```python
from build123d import *

# Parameters (mm, degrees)
SKETCH2_W                = 200
SKETCH2_H                = 150
BOSS_EXTRUDE1_DEPTH      = 80
FILLET1_R                = 10
SHELL1_T                 = -2
SHELL1_THICKNESS_2_DEPTH = 13
SKETCH5_W                = 2
SKETCH5_H                = 4
CUT_EXTRUDE1_DEPTH       = 2
BOSS_EXTRUDE2_DEPTH      = 16
SKETCH7_W                = 36.5
SKETCH7_H                = 27.5
CUT_EXTRUDE2_DEPTH       = 2
BOSS_EXTRUDE3_DEPTH      = 16
SKETCH10_W               = 36.5
SKETCH10_H               = 27.5
CUT_EXTRUDE4_DEPTH       = 2
BOSS_EXTRUDE4_DEPTH      = 16
SKETCH13_W               = 38
SKETCH13_H               = 19.1
CUT_EXTRUDE5_DEPTH       = 2
BOSS_EXTRUDE5_DEPTH      = 13.5
SKETCH15_W               = 10.5
SKETCH15_H               = 9.367949192
CUT_EXTRUDE6_DEPTH       = 3
CUT_EXTRUDE8_REACH       = 150.408
SKETCH20_R               = 8
SPLIT1_SURFACE_1_BACK    = 263.488
SPLIT1_SURFACE_1_DEPTH   = 526.976
SPLIT1_SURFACE_2_BACK    = 263.488
SPLIT1_SURFACE_2_DEPTH   = 526.976
SPLIT2_SURFACE_3_BACK    = 263.488
SPLIT2_SURFACE_3_DEPTH   = 526.976
SPLIT2_SURFACE_4_BACK    = 263.488
SPLIT2_SURFACE_4_DEPTH   = 526.976


with BuildPart() as part:
    # Sketch2 → Boss-Extrude1 (new body)
    with BuildSketch(Plane(origin=(0, 0, 0), x_dir=(1, 0, 0), z_dir=(0, 1, 0))):
        Rectangle(SKETCH2_W, SKETCH2_H)
    extrude(amount=BOSS_EXTRUDE1_DEPTH)

    # Fillet1
    fillet1_edges = [part.edges().sort_by_distance(p)[0] for p in [
        (100, 40, 75),
        (-100, 40, 75),
        (-100, 40, -75),
        (100, 40, -75),
    ]]
    fillet(fillet1_edges, radius=FILLET1_R)

    # Shell1
    shell1_openings = [part.faces().sort_by_distance(p)[0] for p in [
        (0, 80, 0),
    ]]
    offset(amount=SHELL1_T, openings=shell1_openings, kind=Kind.INTERSECTION)

    # Shell1 thickness 2 face (on inner face of the shell) → Shell1 thickness 2 (add)
    with BuildSketch(Plane(origin=(0, 2, 0), x_dir=(0, 0, -1), z_dir=(0, -1, 0))):
        with BuildLine():
            ThreePointArc((73, -90), (70.656854249, -95.656854249), (65, -98))
            Line((65, -98), (-65, -98))
            ThreePointArc((-65, -98), (-70.656854249, -95.656854249), (-73, -90))
            Line((-73, -90), (-73, 90))
            ThreePointArc((-73, 90), (-70.656854249, 95.656854249), (-65, 98))
            Line((-65, 98), (65, 98))
            ThreePointArc((65, 98), (70.656854249, 95.656854249), (73, 90))
            Line((73, 90), (73, -90))
        make_face()
    extrude(amount=-SHELL1_THICKNESS_2_DEPTH)

    # Sketch5 → Cut-Extrude1 (cut)
    with BuildSketch(Plane.XY.offset(75)):
        Polygon((18.25, 44.5), (-18.25, 44.5), (-18.25, 40.5), (-18.25, 21), (-18.25, 17), (18.25, 17), (18.25, 21), (18.25, 40.5), align=None)
        with Locations((-19.25, 42.5)):
            Rectangle(SKETCH5_W, SKETCH5_H)
        with Locations((19.25, 42.5)):
            Rectangle(SKETCH5_W, SKETCH5_H)
        with Locations((-19.25, 19)):
            Rectangle(SKETCH5_W, SKETCH5_H)
        with Locations((19.25, 19)):
            Rectangle(SKETCH5_W, SKETCH5_H)
    extrude(amount=-CUT_EXTRUDE1_DEPTH, mode=Mode.SUBTRACT)

    # Sketch6 → Boss-Extrude2 (add)
    with BuildSketch(Plane(origin=(0, 0, 73), x_dir=(-1, 0, 0), z_dir=(0, 0, -1))):
        Polygon((18.25, 15), (22.25, 15), (22.25, 47.5), (18.25, 47.5), (18.25, 44.5), (20.25, 44.5), (20.25, 40.5), (18.25, 40.5), (18.25, 21), (20.25, 21), (20.25, 17), (18.25, 17), align=None)
        Polygon((-22.25, 47.5), (-22.25, 15), (-18.25, 15), (-18.25, 17), (-20.25, 17), (-20.25, 21), (-18.25, 21), (-18.25, 40.5), (-20.25, 40.5), (-20.25, 44.5), (-18.25, 44.5), (-18.25, 47.5), align=None)
    extrude(amount=BOSS_EXTRUDE2_DEPTH)

    # Sketch7 → Cut-Extrude2 (cut)
    with BuildSketch(Plane(origin=(100, 0, 0), x_dir=(0, 0, -1), z_dir=(1, 0, 0))):
        with Locations((0, 30.75)):
            Rectangle(SKETCH7_W, SKETCH7_H)
        Polygon((-18.25, 43.5), (-19.75, 44.366025404), (-19.75, 41.633974596), (-18.25, 42.5), align=None)
        Polygon((-19.75, 19.866025404), (-18.25, 19), (-18.25, 18), (-19.75, 17.133974596), align=None)
        Polygon((19.75, 17.133974596), (19.75, 19.866025404), (18.25, 19), (18.25, 18), align=None)
        Polygon((19.75, 41.633974596), (18.25, 42.5), (18.25, 43.5), (19.75, 44.366025404), align=None)
    extrude(amount=-CUT_EXTRUDE2_DEPTH, mode=Mode.SUBTRACT)

    # Sketch8 → Boss-Extrude3 (add)
    with BuildSketch(Plane.ZY.offset(-98)):
        Polygon((-21.25, 47.5), (-18.25, 47.5), (-18.25, 43.5), (-19.75, 44.366025404), (-19.75, 41.633974596), (-18.25, 42.5), (-18.25, 19), (-19.75, 19.866025404), (-19.75, 17.133974596), (-18.25, 18), (-18.25, 15), (-21.25, 15), align=None)
        Polygon((19.75, 44.366025404), (18.25, 43.5), (18.25, 47.5), (21.25, 47.5), (21.25, 15), (18.25, 15), (18.25, 18), (19.75, 17.133974596), (19.75, 19.866025404), (18.25, 19), (18.25, 42.5), (19.75, 41.633974596), align=None)
    extrude(amount=BOSS_EXTRUDE3_DEPTH)

    # Sketch10 → Cut-Extrude4 (cut)
    with BuildSketch(Plane.ZY.offset(100)):
        with Locations((0, 30.75)):
            Rectangle(SKETCH10_W, SKETCH10_H)
        Polygon((-18.25, 43.5), (-19.75, 44.366025404), (-19.75, 41.633974596), (-18.25, 42.5), align=None)
        Polygon((-19.75, 19.866025404), (-18.25, 19), (-18.25, 18), (-19.75, 17.133974596), align=None)
        Polygon((19.75, 17.133974596), (19.75, 19.866025404), (18.25, 19), (18.25, 18), align=None)
        Polygon((19.75, 41.633974596), (18.25, 42.5), (18.25, 43.5), (19.75, 44.366025404), align=None)
    extrude(amount=-CUT_EXTRUDE4_DEPTH, mode=Mode.SUBTRACT)

    # Sketch11 → Boss-Extrude4 (add)
    with BuildSketch(Plane(origin=(-98, 0, 0), x_dir=(0, 0, -1), z_dir=(1, 0, 0))):
        Polygon((-18.25, 47.5), (-21.25, 47.5), (-21.25, 15), (-18.25, 15), (-18.25, 18), (-19.75, 17.133974596), (-19.75, 19.866025404), (-18.25, 19), (-18.25, 42.5), (-19.75, 41.633974596), (-19.75, 44.366025404), (-18.25, 43.5), align=None)
        Polygon((19.75, 44.366025404), (18.25, 43.5), (18.25, 47.5), (21.25, 47.5), (21.25, 15), (18.25, 15), (18.25, 18), (19.75, 17.133974596), (19.75, 19.866025404), (18.25, 19), (18.25, 42.5), (19.75, 41.633974596), align=None)
    extrude(amount=BOSS_EXTRUDE4_DEPTH)

    # Sketch13 → Cut-Extrude5 (cut)
    with BuildSketch(Plane.XY.offset(75)):
        Polygon((41, 39.3), (39.5, 40.166025404), (39.5, 37.433974596), (41, 38.3), align=None)
        with Locations((60, 30.75)):
            Rectangle(SKETCH13_W, SKETCH13_H)
        Polygon((41, 22.2), (39.5, 21.333974596), (39.5, 24.066025404), (41, 23.2), align=None)
        Polygon((79, 22.2), (79, 23.2), (80.5, 24.066025404), (80.5, 21.333974596), align=None)
        Polygon((79, 39.3), (80.5, 40.166025404), (80.5, 37.433974596), (79, 38.3), align=None)
    extrude(amount=-CUT_EXTRUDE5_DEPTH, mode=Mode.SUBTRACT)

    # Sketch14 → Boss-Extrude5 (add)
    with BuildSketch(Plane(origin=(0, 0, 73), x_dir=(-1, 0, 0), z_dir=(0, 0, -1))):
        Polygon((-79, 43.3), (-82, 43.3), (-82, 15), (-79, 15), (-79, 22.2), (-80.5, 21.333974596), (-80.5, 24.066025404), (-79, 23.2), (-79, 38.3), (-80.5, 37.433974596), (-80.5, 40.166025404), (-79, 39.3), align=None)
        Polygon((-39.5, 40.166025404), (-41, 39.3), (-41, 43.3), (-38, 43.3), (-38, 15), (-41, 15), (-41, 22.2), (-39.5, 21.333974596), (-39.5, 24.066025404), (-41, 23.2), (-41, 38.3), (-39.5, 37.433974596), align=None)
    extrude(amount=BOSS_EXTRUDE5_DEPTH)

    # Sketch15 → Cut-Extrude6 (cut)
    with BuildSketch(Plane.ZY.offset(-38)):
        with Locations((66.75, 30.75)):
            Rectangle(SKETCH15_W, SKETCH15_H)
    extrude(amount=-CUT_EXTRUDE6_DEPTH, mode=Mode.SUBTRACT)

    # Sketch18 → Cut-Revolve1 (revolve, cut)
    with BuildSketch(Plane(origin=(0, 0, 0), x_dir=(0, 0, -1), z_dir=(1, 0, 0)), mode=Mode.PRIVATE) as cut_revolve1_sk:
        Polygon((-42.5, 0), (-70, 0), (-47.5, 10), (-42.5, 10), align=None)
    revolve(cut_revolve1_sk.sketch.rotate(Axis((0, 0, 0), (0, 1, 0)), 180), axis=Axis((0, 0, 0), (0, 1, 0)), mode=Mode.SUBTRACT)

    # Cut-Extrude8: up to this face of the body (flat: up to its plane)
    cut_extrude8_end = Plane(part.part.faces().sort_by_distance((-0.172584848, 15, -0.486016332))[0])
    # Sketch20 → Cut-Extrude8 (cut, up to the picked face)
    with BuildSketch(Plane.XZ, mode=Mode.PRIVATE) as cut_extrude8_sk1:
        with Locations(Location((0, -42.5, 0), (0, 0, 270))):
            Circle(SKETCH20_R)
    cut_extrude8_tool1 = split(extrude(cut_extrude8_sk1.sketch, amount=-CUT_EXTRUDE8_REACH, mode=Mode.PRIVATE), bisect_by=cut_extrude8_end, keep=Keep.BOTH, mode=Mode.PRIVATE)
    add(cut_extrude8_tool1.solids().sort_by(Axis((0, 0, -42.5), (0, 1, 0)))[0], mode=Mode.SUBTRACT)


with BuildPart() as body_2:
    # Split1: the piece behind the surface
    add(part.part)
    # Split1 surface: a surface, the sketch's curves swept straight by 526.976 mm
    with BuildLine(Plane.XY.offset(75).offset(-SPLIT1_SURFACE_1_BACK), mode=Mode.PRIVATE) as split1_surface_1_path:
        Line((-23.25, 49.5), (23.25, 49.5))
        Line((23.25, 49.5), (23.25, 12))
        Line((23.25, 12), (-23.25, 12))
        Line((-23.25, 12), (-23.25, 49.5))
    split1_surface_1 = Shell.extrude(split1_surface_1_path.wire(), (0 * SPLIT1_SURFACE_1_DEPTH, 0 * SPLIT1_SURFACE_1_DEPTH, 1 * SPLIT1_SURFACE_1_DEPTH))
    split(bisect_by=split1_surface_1, keep=Keep.BOTTOM)


with BuildPart() as part_1:
    add(part.part)

    # Split1: split by a surface, the side it looks to stays
    # Split1 surface: a surface, the sketch's curves swept straight by 526.976 mm
    with BuildLine(Plane.XY.offset(75).offset(-SPLIT1_SURFACE_2_BACK), mode=Mode.PRIVATE) as split1_surface_2_path:
        Line((-23.25, 49.5), (23.25, 49.5))
        Line((23.25, 49.5), (23.25, 12))
        Line((23.25, 12), (-23.25, 12))
        Line((-23.25, 12), (-23.25, 49.5))
    split1_surface_2 = Shell.extrude(split1_surface_2_path.wire(), (0 * SPLIT1_SURFACE_2_DEPTH, 0 * SPLIT1_SURFACE_2_DEPTH, 1 * SPLIT1_SURFACE_2_DEPTH))
    split(bisect_by=split1_surface_2, keep=Keep.TOP)


with BuildPart() as body_3:
    # Split2: the piece behind the surface
    add(body_2.part)
    # Split2 surface: a surface, the sketch's curves swept straight by 526.976 mm
    with BuildLine(Plane(origin=(0, 15, 0), x_dir=(1, 0, 0), z_dir=(0, 1, 0)).offset(-SPLIT2_SURFACE_3_BACK), mode=Mode.PRIVATE) as split2_surface_3_path:
        Line((-23.25, -75), (23.25, -75))
        Line((23.25, -75), (23.25, -50))
        Line((23.25, -50), (-23.25, -50))
        Line((-23.25, -50), (-23.25, -75))
    split2_surface_3 = Shell.extrude(split2_surface_3_path.wire(), (0 * SPLIT2_SURFACE_3_DEPTH, 1 * SPLIT2_SURFACE_3_DEPTH, 0 * SPLIT2_SURFACE_3_DEPTH))
    split(bisect_by=split2_surface_3, keep=Keep.BOTTOM)


with BuildPart() as body_2_1:
    add(body_2.part)

    # Split2: split by a surface, the side it looks to stays
    # Split2 surface: a surface, the sketch's curves swept straight by 526.976 mm
    with BuildLine(Plane(origin=(0, 15, 0), x_dir=(1, 0, 0), z_dir=(0, 1, 0)).offset(-SPLIT2_SURFACE_4_BACK), mode=Mode.PRIVATE) as split2_surface_4_path:
        Line((-23.25, -75), (23.25, -75))
        Line((23.25, -75), (23.25, -50))
        Line((23.25, -50), (-23.25, -50))
        Line((-23.25, -50), (-23.25, -75))
    split2_surface_4 = Shell.extrude(split2_surface_4_path.wire(), (0 * SPLIT2_SURFACE_4_DEPTH, 1 * SPLIT2_SURFACE_4_DEPTH, 0 * SPLIT2_SURFACE_4_DEPTH))
    split(bisect_by=split2_surface_4, keep=Keep.TOP)


solid = body_2_1.part
```
Design review of the part built by this model. Coordinates are the model's own, in mm. A direction names the side the tool comes from. Give positions to 0.01 mm unless a question says otherwise; leave off trailing zeros. Write each loop counter-clockwise with the first axis right and the second up, starting at its lowest first coordinate (ties: lowest second). Pieces come first, ordered by that corner, then holes.
(1) Add section D-D (z = 54.25). Give the boundary of the cut face in (x, y).
Checked values:
outline: (-23.25, 12) - (23.25, 12) - (23.25, 15) - (-23.25, 15) - close
(2) Wall thickness on line 1 along Y through (x, z) = (-19.5, 68); line 2 along X through (y, z) = (40, 72); line 3 along X through (y, z) = (42, 70.75): over which ranges is each line inside the solid? List them lowest first.
Checked values:
line 1: y = 12 to 17, 21 to 40.5, 44.5 to 47.5
line 2: x = -22.25 to -18.25, 18.25 to 22.25
line 3: x = -22.25 to -20.25, 20.25 to 22.25
(3) Add section A-A (y = 29). Give the boundary of the cut face in (x, z).
Checked values:
outline: (-23.25, 73) - (-22.25, 73) - (-22.25, 57) - (-18.25, 57) - (-18.25, 75) - (-23.25, 75) - close; (18.25, 57) - (22.25, 57) - (22.25, 73) - (23.25, 73) - (23.25, 75) - (18.25, 75) - close
(4) Add section B-B (x = -3). Give the boundary of the cut face in (y, z), and give its area (3 significant figures).
Checked values:
outline: (12, 50) - (15, 50) - (15, 73) - (17, 73) - (17, 75) - (12, 75) - close; (44.5, 73) - (49.5, 73) - (49.5, 75) - (44.5, 75) - close
area: 89.0 mm2
(5) Tool access review of faces 1 (the face through (20.25, 42, 66)), 2 (the face through (-18.25, 16, 65)), 3 (the face through (-22.25, 31, 65)): name each direction out of +Z, -Z, +X, -X, +Y, -Y from which nothing blocks a thin tool from reaching the whole face with its end or side.
Checked values:
face 1: +Z, -Z
face 2: -Z, +Y
face 3: -Z, -X, +Y
(6) Clearance check with flat-ended pins moving along their axes: pin 1 Ø1.2 at (x, z) = (-20.5, 61) entering from +Y; pin 2 Ø1.5 at (x, y) = (-2, 42.5) entering from +Z; pin 3 Ø3 at (y, z) = (39, 56.5) entering from +X; pin 4 Ø4 at (x, z) = (10.5, 63.5) entering from +Y. State where each tip first meets the part, or that it passes through.
Checked values:
pin 1: stops at y = 47.5
pin 2: passes through
pin 3: stops at x = 22.25
pin 4: stops at y = 15
(7) Mouldability with a two-part tool opening along X and no side actions: class faces 4 (the face through (-20.25, 43, 66)), 5 (the face through (0, 49.5, 74)), 6 (the face through (23.25, 23, 74)) as +X half, -X half, draft (parallel to the pull), parting line (faces both ways), or undercut.
Checked values:
face 4: undercut
face 5: draft
face 6: +X half
(8) Add section C-C (z = 61). Give the boundary of the cut face in (x, y).
Checked values:
outline: (-23.25, 12) - (23.25, 12) - (23.25, 15) - (22.25, 15) - (22.25, 47.5) - (18.25, 47.5) - (18.25, 44.5) - (20.25, 44.5) - (20.25, 40.5) - (18.25, 40.5) - (18.25, 21) - (20.25, 21) - (20.25, 17) - (18.25, 17) - (18.25, 15) - (-18.25, 15) - (-18.25, 17) - (-20.25, 17) - (-20.25, 21) - (-18.25, 21) - (-18.25, 40.5) - (-20.25, 40.5) - (-20.25, 44.5) - (-18.25, 44.5) - (-18.25, 47.5) - (-22.25, 47.5) - (-22.25, 15) - (-23.25, 15) - close
